Autodesk Fusion 360 part; units mm, degrees
sketch "Sketch1" plane through (0, 0, 0) normal (0, 0, 1) x (1, 0, 0)
  circle A0 centre (0, 0) radius 20
  line L0 (4.0415, 0) -> (2.0207, 3.5)
  line L1 (2.0207, 3.5) -> (-2.0207, 3.5)
  line L2 (-2.0207, 3.5) -> (-4.0415, 0)
  line L3 (-4.0415, 0) -> (-2.0207, -3.5)
  line L4 (-2.0207, -3.5) -> (2.0207, -3.5)
  line L5 (2.0207, -3.5) -> (4.0415, 0)
  dimension "d1" = 40
  dimension "d10" = 7
extrude "Extrude1" add sketch "Sketch1" along normal blind 2
sketch "Sketch2" plane through (0, 0, 2) normal (0, 0, 1) x (-1, 0, 0)
  circle A0 centre (0, 0) radius 20
  circle A1 centre (0, 0) radius 8
  line L0 (-4.0415, 0) -> (-2.0207, 3.5)
  line L1 (-2.0207, 3.5) -> (2.0207, 3.5)
  line L2 (2.0207, 3.5) -> (4.0415, 0)
  line L3 (4.0415, 0) -> (2.0207, -3.5)
  line L4 (2.0207, -3.5) -> (-2.0207, -3.5)
  line L5 (-2.0207, -3.5) -> (-4.0415, 0)
  dimension "d4" = 16
extrude "Extrude2" add sketch "Sketch2" along normal blind 0.3 contours A1
sketch "Sketch3" plane through (0, 0, 2.3) normal (0, 0, 1) x (-1, 0, 0)
  circle A0 centre (0, 0) radius 8
  circle A1 centre (0, 0) radius 6
  line L0 (2.0207, -3.5) -> (-2.0207, -3.5)
  line L1 (-2.0207, -3.5) -> (-4.0415, 0)
  line L2 (-4.0415, 0) -> (-2.0207, 3.5)
  line L3 (-2.0207, 3.5) -> (2.0207, 3.5)
  line L4 (2.0207, 3.5) -> (4.0415, 0)
  line L5 (4.0415, 0) -> (2.0207, -3.5)
  dimension "d7" = 12
extrude "Extrude3" add sketch "Sketch3" along normal blind 3.5 contours A1
Source: CAD feature listing. Evaluate the final solid. Frame: model axes, mm. A direction names the side the tool comes from. Give positions to 0.01 mm unless a question says otherwise; leave off trailing zeros. Write each loop counter-clockwise with the first axis right and the second up, starting at its lowest first coordinate (ties: lowest second). Pieces come first, ordered by that corner, then holes. Notation, with made-up numbers: M 70,46.25 L 109,46.25 A12 cw 109,56.25 Z; hole C 4.5,-28.75 d4. An arc over 180 degrees is marked long. Return JSON: item names as keys, results as strings. Group by question number.
1) Set-up query: faces 4 (the face through (6, 0, 4)), 5 (the face through (3, 1.8, 2.9)), 6 (the face through (4.2, 0.3, 0)). Return all of +Z, -Z, +X, -X, +Y, -Y with unobstructed straight access to the full face (end or side cutting, diameter ignored); none if empty.
2) Cut plane C-C, the plane y = 3. Output: boundary loops of the cut face in (x, z), plus the area to 3 significant figures.
3) Cut plane D-D, the plane z = 5.15. Output: boundary loops of the cut face in (x, y).
4) Pull-direction query (X, two-part tool) for faces 1 (the face through (2, -6, 2.3)), 2 (the face through (-4.336, 19.524, 0.986)), 3 (the face through (-3.045, 1.726, 2.859)); classes: pulls with the +X half, pulls with the -X half, needs draft (parallel to the pull), parting line crosses it, or undercut.
5) Cut plane A-A, the plane x = 0. Output: boundary loops of the cut face in (y, z).
6) Pin query (flat end, axial travel): P1, Ø1, axis at x = 6.5, z = 2, coming from the +Y side; P2, Ø1, axis at x = -12, z = 1.5, coming from the +Y side; P3, Ø3, axis at y = 15.5, z = 0.5, coming from the -X side. Return the tip coordinate at first contact, or that it passes through.
7) Material intervals for line 1 along Z through (x, y) = (-7.5, 7.5); line 2 along Z through (x, y) = (-7, -2.5); line 3 along Y through (x, z) = (1, 4.55), sorted ascending. Write a range as [from, to].
8) Cut plane B-B, the plane z = 0.9. Output: boundary loops of the cut face in (x, y).
Recorded:
{
 "1": {"face 4": "+Z", "face 5": "+Z, -Z", "face 6": "-Z, +X, -X, +Y, -Y"},
 "2": {"outline": "M -19.77,0 L -2.31,0 L -2.31,5.8 L -5.2,5.8 L -5.2,2.3 L -7.42,2.3 L -7.42,2 L -19.77,2 Z; M 2.31,0 L 19.77,0 L 19.77,2 L 7.42,2 L 7.42,2.3 L 5.2,2.3 L 5.2,5.8 L 2.31,5.8 Z", "area": "93.1 mm²"},
 "3": {"outline": "C 0,0 d12; hole M -4.04,0 L -2.02,-3.5 L 2.02,-3.5 L 4.04,0 L 2.02,3.5 L -2.02,3.5 Z"},
 "4": {"face 1": "needs draft", "face 2": "parting line crosses it", "face 3": "undercut"},
 "5": {"outline": "M -20,0 L -3.5,0 L -3.5,5.8 L -6,5.8 L -6,2.3 L -8,2.3 L -8,2 L -20,2 Z; M 3.5,0 L 20,0 L 20,2 L 8,2 L 8,2.3 L 6,2.3 L 6,5.8 L 3.5,5.8 Z"},
 "6": {"P1": "stops at y = 19.08", "P2": "stops at y = 16.36", "P3": "stops at x = -14.28"},
 "7": {"line 1": "z = [0, 2]", "line 2": "z = [0, 2.3]", "line 3": "y = [-5.92, -3.5], [3.5, 5.92]"},
 "8": {"outline": "C 0,0 d40; hole M -4.04,0 L -2.02,-3.5 L 2.02,-3.5 L 4.04,0 L 2.02,3.5 L -2.02,3.5 Z"}
}
